Autodesk Inventor part; units mm, degrees
ref_plane "YZ Plane" through (0, 0, 0) normal (1, 0, 0) x (0, 1, 0)
ref_plane "XZ Plane" through (0, 0, 0) normal (0, 1, 0) x (-1, 0, 0)
ref_plane "XY Plane" through (0, 0, 0) normal (0, 0, 1) x (1, 0, 0)
sketch "草图1" plane through (0, 0, 0) normal (0, 1, 0) x (-1, 0, 0)
  line L0 (0, 0) -> (-195, 0)
  line L1 (-195, 0) -> (-195, -315)
  line L2 (-195, -315) -> (0, -315)
  line L3 (0, -315) -> (0, 0)
  dimension "d0" = 195
  dimension "d1" = 315
extrude "拉伸1" add sketch "草图1" along normal blind 13
shell "抽壳1" thickness 2 removed faces 1 at (65, 13, -210)
chamfer "倒角1" distance 2 angle 45 8 edges at (97.5, 0, 0) (0, 0, -157.5) (195, 0, -157.5) (97.5, 0, -315) (195, 6.5, -315) (195, 6.5, 0) (0, 6.5, 0) (0, 6.5, -315)
properties part number "test"
Here's how the part is built. I have some questions about the finished solid (model axes, mm). A direction names the side the tool comes from. Round coordinates to 2 decimals unless told otherwise and drop trailing zeros. Loops run counter-clockwise (first coordinate to the right, second up) from the corner with the lowest first, then second, coordinate; pieces in that order, holes last. Notation, with made-up numbers: (55, 38.25) - (110, 38.25) arc R17 cw to (110, 61.25) - close; hole circle Ø3 at (35, -24). An arc over 180 degrees is marked (long way). One line per question, with ' | ' between items. Start each with the question number.
Q1. Will these pins go through, and if not, where does the flat tip stop? pin 1 (1 mm diameter, centred on x = 74, z = -154.5, fed in from +Y); pin 2 (6 mm diameter, centred on x = 41.5, y = 10, fed in from +Z).
Q2. Please list where these lines run through material, in increasing order: line 1 (Z direction, x = 179, y = 8); line 2 (X direction, y = 9.75, z = -27.5); line 3 (Y direction, x = 118, z = -258.5). Write a range as [from, to].
Q3. For faces 1 (the flat face through (99, 0, -155)), 2 (the flat face through (96, 7, -2)), which set-ups out of +Z, -Z, +X, -X, +Y, -Y let a thin tool reach every point of the face, with its end or its side?
Q4. I want a section at A-A (y = 10). Write out the boundary of the cut face in (x, z).
Q5. I want a section at C-C (z = -83). Write out the boundary of the cut face in (x, y), then the cut area to 3 significant figures.
Q6. We'd pull the mould along X, two halves only. Please class faces 3 (the flat face through (193, 7, -155)), 4 (the flat face through (99, 7, -315)), 5 (the flat face through (0, 7, -160)): +X half, -X half, draft (parallel to the pull), parting line (faces both ways), or undercut.
Q7. I want a section at B-B (x = 167.5). Write out the boundary of the cut face in (y, z).
Response values:
1) pin 1: stops at y = 2 | pin 2: stops at z = 0
2) line 1: z = [-315, -313], [-2, 0] | line 2: x = [0, 2], [193, 195] | line 3: y = [0, 2]
3) face 1: +Z, -Z, +X, -X, -Y | face 2: +Y
4) outline: (0, -313) - (2, -315) - (193, -315) - (195, -313) - (195, -2) - (193, 0) - (2, 0) - (0, -2) - close; hole (2, -313) - (193, -313) - (193, -2) - (2, -2) - close
5) outline: (0, 2) - (2, 0) - (193, 0) - (195, 2) - (195, 13) - (193, 13) - (193, 2) - (2, 2) - (2, 13) - (0, 13) - close | area: 430 mm²
6) face 3: undercut | face 4: draft | face 5: -X half
7) outline: (0, -313) - (2, -315) - (13, -315) - (13, -313) - (2, -313) - (2, -2) - (13, -2) - (13, 0) - (2, 0) - (0, -2) - close
